from build123d import *

# Parameters (mm, degrees)
BOSS_EXTRUDE1_DEPTH = 3.048


with BuildPart() as part:
    # Sketch1 → Boss-Extrude1 (new, symmetric)
    with BuildSketch(Plane(origin=(0, 0, 0), x_dir=(1, 0, 0), z_dir=(0, 1, 0))):
        with BuildLine():
            Line((-49.53, 45.72), (49.53, 45.72))
            Line((49.53, 45.72), (49.53, 38.1))
            Line((49.53, 38.1), (55.626, 38.1))
            Line((55.626, 38.1), (55.626, -8.951856626))
            Line((55.626, -8.951856626), (49.53, -8.951856626))
            Line((49.53, -8.951856626), (49.53, -16.571856626))
            Line((49.53, -16.571856626), (55.626, -16.571856626))
            Line((55.626, -16.571856626), (55.626, -29.271856626))
            Line((55.626, -29.271856626), (21.019827136, -42.136821893))
            ThreePointArc((21.019827136, -42.136821893), (17.95098831, -44.911778638), (17.631953735, -49.036869377))
            Line((17.631953735, -49.036869377), (25.187729856, -73.287029113))
            ThreePointArc((25.187729856, -73.287029113), (26.234780075, -75.207903536), (27.939063878, -76.579577488))
            ThreePointArc((27.939063878, -76.579577488), (41.468907088, -82.632484358), (55.626, -87.022365809))
            Line((55.626, -87.022365809), (55.626, -132.617292876))
            Line((55.626, -132.617292876), (-49.53, -132.617292876))
            Line((-49.53, -132.617292876), (-49.53, -124.997292876))
            Line((-49.53, -124.997292876), (-55.626, -124.997292876))
            Line((-55.626, -124.997292876), (-55.626, -97.057292876))
            Line((-55.626, -97.057292876), (-49.53, -97.057292876))
            Line((-49.53, -97.057292876), (-49.53, -85.359826344))
            ThreePointArc((-49.53, -85.359826344), (-38.527111219, -81.479756652), (-27.939063878, -76.579577488))
            ThreePointArc((-27.939063878, -76.579577488), (-26.234780075, -75.207903536), (-25.187729856, -73.287029113))
            Line((-25.187729856, -73.287029113), (-17.631953735, -49.036869377))
            ThreePointArc((-17.631953735, -49.036869377), (-17.95098831, -44.911778638), (-21.019827136, -42.136821893))
            Line((-21.019827136, -42.136821893), (-55.626, -29.271856626))
            Line((-55.626, -29.271856626), (-55.626, -16.571856626))
            Line((-55.626, -16.571856626), (-49.53, -16.571856626))
            Line((-49.53, -16.571856626), (-49.53, -8.951856626))
            Line((-49.53, -8.951856626), (-55.626, -8.951856626))
            Line((-55.626, -8.951856626), (-55.626, 38.1))
            Line((-55.626, 38.1), (-49.53, 38.1))
            Line((-49.53, 38.1), (-49.53, 45.72))
        make_face()
    extrude(amount=BOSS_EXTRUDE1_DEPTH, both=True)


solid = part.part
Here's how the part is built. I have some questions about the finished solid (model axes, mm). A direction names the side the tool comes from. Give positions to 0.01 mm unless a question says otherwise; leave off trailing zeros. Order: outer loops, then holes, each group sorted by start corner. A loop starts at its lowest first (then second) coordinate and runs counter-clockwise, first axis right, second up. Notation, with made-up numbers: M 74.5,24.5 L 92.5,24.5 A12 ccw 92.5,39.5 Z; hole C 30,81.5 d2. An arc over 180 degrees is marked long. Answer as a JSON object with one key per item and string values. Group by question number.
1) Suppose I cut it at D-D, the plane z = 89.5. Write out the boundary of the cut face in (x, y), plus the area to 3 significant figures.
2) We'd pull the mould along Z, two halves only. Please class faces 6 (the flat face through (1, -3.048, 42)), 7 (the flat face through (-53, 0, 97.057)), 8 (the flat face through (-1, 0, -45.72)): pulls with the +Z half, pulls with the -Z half, needs draft (parallel to the pull), parting line crosses it, or undercut.
3) Suppose I cut it at A-A, the plane x = 35. Write out the boundary of the cut face in (y, z), plus the area to 3 significant figures.
4) Suppose I cut it at C-C, the plane x = -23. Write out the boundary of the cut face in (y, z).
5) Please list where these lines run through material, in increasing order: L1, parallel to Z at x = -39, y = 1.75; L2, parallel to Z at x = 48, y = -0.5; L3, parallel to X at y = -2, z = 14. Write a range as [from, to].
6) I'm going to push flat-ended pins straight in: pin 1 Ø1.8 at (x, y) = (-52.5, 1.5) entering from -Z; pin 2 Ø1.8 at (x, y) = (-53, 1) entering from +Z; pin 3 Ø3 at (y, z) = (1, 11) entering from -X. Where does each tip first touch, or does it pass through?
7) On a 3-axis mill with a long thin cutter (end or side, diameter ignored), from which of +Z, -Z, +X, -X, +Y, -Y can I reach the whole of each face in a straight line? I mean faces 1 (the flat face through (-49.53, 0, 129)), 2 (the flat face through (38.6, 0, 35.6)), 3 (the flat face through (-49.53, 0, 91)), 4 (the flat face through (53, 0, -38.1)), 5 (the flat face through (-53, 0, -38.1)). Say none if no direction works.
Results found:
{
 "1": {"outline": "M -49.53,-3.05 L 55.63,-3.05 L 55.63,3.05 L -49.53,3.05 Z", "area": "641 mm²"},
 "2": {"face 6": "needs draft", "face 7": "undercut", "face 8": "pulls with the -Z half"},
 "3": {"outline": "M -3.05,-45.72 L 3.05,-45.72 L 3.05,36.94 L -3.05,36.94 Z; M -3.05,79.98 L 3.05,79.98 L 3.05,132.62 L -3.05,132.62 Z", "area": "825 mm²"},
 "4": {"outline": "M -3.05,-45.72 L 3.05,-45.72 L 3.05,41.4 L -3.05,41.4 Z; M -3.05,66.27 L 3.05,66.27 L 3.05,132.62 L -3.05,132.62 Z"},
 "5": {"L1": "[-45.72, 35.45], [81.67, 132.62]", "L2": "[-45.72, 32.11], [84.89, 132.62]", "L3": "[-49.53, 49.53]"},
 "6": {"pin 1": "z = -38.1", "pin 2": "z = 125", "pin 3": "x = -49.53"},
 "7": {"face 1": "+Z, -X, +Y, -Y", "face 2": "+X, +Y, -Y", "face 3": "-X, +Y, -Y", "face 4": "-Z, +X, +Y, -Y", "face 5": "-Z, -X, +Y, -Y"}
}
